Could you check a few things on this model? Use its own coordinates, in mm. Face numbers are marked on the shaded views. Give positions to 0.01 mm unless a question says otherwise; leave off trailing zeros. Write each loop counter-clockwise with the first axis right and the second up, starting at its lowest first coordinate (ties: lowest second). Pieces come first, ordered by that corner, then holes. Notation, with made-up numbers: (22.5, 47) - (70.5, 47) arc R26 cw to (70.5, 75) - close; hole circle Ø4 at (79.25, 75). An arc over 180 degrees is marked (long way). Answer in a Markdown table with one row per item.
from build123d import *

# Parameters (mm, degrees)
SKETCH1_W           = 118.11
SKETCH1_H           = 80.01
BOSS_EXTRUDE1_DEPTH = 12.7
SKETCH2_R           = 4.445
CUT_EXTRUDE1_DEPTH  = 13.7
SKETCH3_R           = 7.9375
CUT_EXTRUDE2_DEPTH  = 13.7


with BuildPart() as part:
    # Sketch1 → Boss-Extrude1 (new body)
    with BuildSketch(Plane(origin=(0, 0, 0), x_dir=(1, 0, 0), z_dir=(0, 1, 0))):
        Rectangle(SKETCH1_W, SKETCH1_H)
    extrude(amount=BOSS_EXTRUDE1_DEPTH)

    # Sketch2 → Cut-Extrude1 (cut, through all)
    with BuildSketch(Plane.XZ):
        with Locations((-30.00502, 30.00502)):
            Circle(SKETCH2_R)
        with Locations((30.00502, 30.00502)):
            Circle(SKETCH2_R)
        with Locations((-30.00502, -30.00502)):
            Circle(SKETCH2_R)
        with Locations((30.00502, -30.00502)):
            Circle(SKETCH2_R)
    extrude(amount=-CUT_EXTRUDE1_DEPTH, mode=Mode.SUBTRACT)

    # Sketch3 → Cut-Extrude2 (cut, through all)
    with BuildSketch(Plane.XZ):
        with Locations((-49.53, 27.305)):
            Circle(SKETCH3_R)
        with Locations((-49.53, -27.305)):
            Circle(SKETCH3_R)
        with Locations((49.53, -27.305)):
            Circle(SKETCH3_R)
        with Locations((49.53, 27.305)):
            Circle(SKETCH3_R)
    extrude(amount=-CUT_EXTRUDE2_DEPTH, mode=Mode.SUBTRACT)


solid = part.part
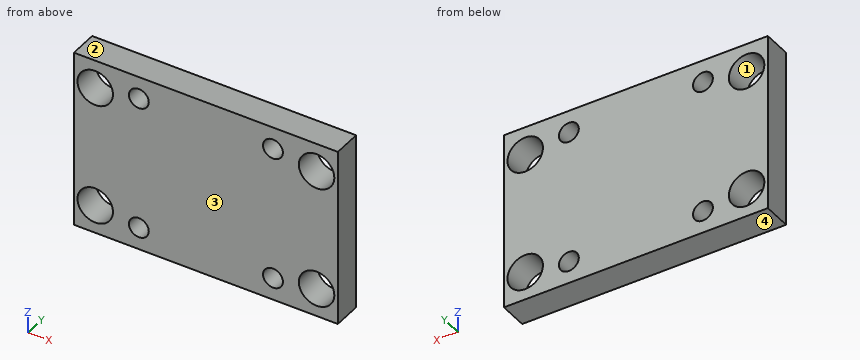
1) We'd pull the mould along Z, two halves only. Please class the marked faces 1, 2, 3 and 4: +Z half, -Z half, draft (parallel to the pull), parting line (faces both ways), or undercut.
Check values:
| item | result |
|---|---|
| face 1 | undercut |
| face 2 | +Z half |
| face 3 | draft |
| face 4 | -Z half |
2) Imagine slicing it at C-C (x = -28.5). List the corners of the cut face in (y, z) for me (3 decimals).
Check values:
| item | result |
|---|---|
| outline | (0, -40.005) - (12.7, -40.005) - (12.7, -34.187) - (0, -34.187) - close; (0, -25.823) - (12.7, -25.823) - (12.7, 25.823) - (0, 25.823) - close; (0, 34.187) - (12.7, 34.187) - (12.7, 40.005) - (0, 40.005) - close |
3) If I drill on line 1 (Z direction, x = -49.53, y = 6.5) (1 decimal); line 2 (X direction, y = 3.5, z = 29) (3 decimals); line 3 (X direction, y = 7.25, z = 22) (3 decimals), over which ranges is the centre line in solid material (lowest first)?
Check values:
| item | result |
|---|---|
| line 1 | z = -40 to -35.2, -19.4 to 19.4, 35.2 to 40 |
| line 2 | x = -59.055 to -57.284, -41.776 to -34.335, -25.675 to 25.675, 34.335 to 41.776, 57.284 to 59.055 |
| line 3 | x = -59.055 to -55.434, -43.626 to 43.626, 55.434 to 59.055 |
4) Imagine slicing it at A-A (x = -49.53). List the corners of the cut face in (y, z) for me (1 decimal).
Check values:
| item | result |
|---|---|
| outline | (0, -40) - (12.7, -40) - (12.7, -35.2) - (0, -35.2) - close; (0, -19.4) - (12.7, -19.4) - (12.7, 19.4) - (0, 19.4) - close; (0, 35.2) - (12.7, 35.2) - (12.7, 40) - (0, 40) - close |
5) Imagine slicing it at B-B (y = 8). State how many separate pieces and enclosed holes the cut face has, then the cut area to 3 significant figures.
Check values:
| item | result |
|---|---|
| separate pieces | 1 |
| enclosed holes | 8 |
| area | 8,410 mm2 |
6) Will these pins go through, and if not, where does the flat tip stop? P1, Ø8, axis at x = -30.01, z = -30.01, coming from the -Y side; P2, Ø18.5, axis at x = 49.53, z = 27.305, coming from the -Y side.
Check values:
| item | result |
|---|---|
| P1 | passes through |
| P2 | stops at y = 0 |
